The model under review builds one solid part; all positions refer to its coordinate system, in mm. Face numbers are marked on the shaded views. A direction names the side the tool comes from. Give positions to 0.01 mm unless a question says otherwise; leave off trailing zeros. Order: outer loops, then holes, each group sorted by start corner. A loop starts at its lowest first (then second) coordinate and runs counter-clockwise, first axis right, second up. Notation, with made-up numbers: (70.25, -40) - (114.25, -40) arc R13 cw to (114.25, -24) - close; hole circle Ø11 at (-12, 77.5). An arc over 180 degrees is marked (long way). Use CSV: the item, a comma, the result in double quotes. Start each with the question number.
1. Machinability: for the marked faces 1 and 2, which of the approach directions +Z, -Z, +X, -X, +Y, -Y give a long, thin tool a straight path to every point of the face, cutting with its end or side? Answer none if there is none.
2. Take a section at A-A, the plane x = 0. State the section outline as (y, z) points.
3. For pin 1 (2 mm diameter, centred on y = 4, z = 2, fed in from +X), flat-tipped, find the tip position at first contact; note if it passes through.
4. Take a section at D-D, the plane y = 4.85. State the section outline as (x, z) points, then the cut area to 3 significant figures.
5. To check wall thickness, follow line 1 (Y direction, x = 1.25, z = 2.5); line 2 (X direction, y = 4.3, z = 0). State the ranges of each line that lie inside material, in increasing order. Write a range as [from, to].
6. Take a section at C-C, the plane z = 0. State the section outline as (x, y) points.
7. Take a section at B-B, the plane y = 1.7. State the section outline as (x, z) points.
8. Draft analysis for pull direction Z (two halves, no side actions). For the marked faces 3, 4 and 5, state which applies: released by +Z, released by -Z, zero draft, split by the parting line, or undercut.
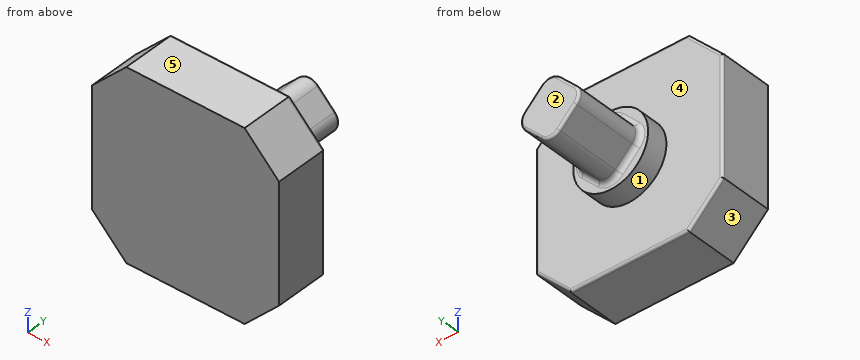
```python
from build123d import *

# Parameters (mm, degrees)
BOSS_EXTRUDE1_DEPTH = 2.14
FILLET1_R           = 0.1
SKETCH2_R           = 1.5
BOSS_EXTRUDE2_DEPTH = 0.86
BOSS_EXTRUDE3_DEPTH = 2.86
FILLET2_R           = 0.1
FILLET3_R           = 0.2


with BuildPart() as part:
    # Sketch1 → Boss-Extrude1 (new body)
    with BuildSketch(Plane(origin=(0, 0, 0), x_dir=(1, 0, 0), z_dir=(0, 1, 0))):
        Polygon((2.371141777, -3.75), (3.75, -2.371141777), (3.75, 2.371141777), (2.371141777, 3.75), (-2.371141777, 3.75), (-3.75, 2.371141777), (-3.75, -2.371141777), (-2.371141777, -3.75), align=None)
    extrude(amount=BOSS_EXTRUDE1_DEPTH)

    # Fillet1
    fillet1_edges = [part.edges().sort_by_distance(p)[0] for p in [
        (3.75, 2.14, 0),
        (3.060570888, 2.14, -3.060570888),
        (0, 2.14, -3.75),
        (-3.060570888, 2.14, -3.060570888),
        (-3.75, 2.14, 0),
        (-3.060570888, 2.14, 3.060570888),
        (0, 2.14, 3.75),
        (3.060570888, 2.14, 3.060570888),
    ]]
    fillet(fillet1_edges, radius=FILLET1_R)

    # Sketch2 → Boss-Extrude2 (add)
    with BuildSketch(Plane(origin=(0, 2.14, 0), x_dir=(1, 0, 0), z_dir=(0, 1, 0))):
        Circle(SKETCH2_R)
    extrude(amount=BOSS_EXTRUDE2_DEPTH)

    # Sketch3 → Boss-Extrude3 (add)
    with BuildSketch(Plane(origin=(0, 3, 0), x_dir=(1, 0, 0), z_dir=(0, 1, 0))):
        with BuildLine():
            Line((-0.353553391, 1.025304833), (-1.025304833, 0.353553391))
            ThreePointArc((-1.025304833, 0.353553391), (-1.171751442, 0), (-1.025304833, -0.353553391))
            Line((-1.025304833, -0.353553391), (-0.353553391, -1.025304833))
            ThreePointArc((-0.353553391, -1.025304833), (0, -1.171751442), (0.353553391, -1.025304833))
            Line((0.353553391, -1.025304833), (1.025304833, -0.353553391))
            ThreePointArc((1.025304833, -0.353553391), (1.171751442, 0), (1.025304833, 0.353553391))
            Line((1.025304833, 0.353553391), (0.353553391, 1.025304833))
            ThreePointArc((0.353553391, 1.025304833), (0, 1.171751442), (-0.353553391, 1.025304833))
        make_face()
    extrude(amount=BOSS_EXTRUDE3_DEPTH)

    # Fillet2
    fillet2_edges = [part.edges().sort_by_distance(p)[0] for p in [
        (-1.171751442, 5.86, 0),
        (-0.689429112, 5.86, 0.689429112),
        (0, 5.86, 1.171751442),
        (0.689429112, 5.86, 0.689429112),
        (1.171751442, 5.86, 0),
        (0.689429112, 5.86, -0.689429112),
        (0, 5.86, -1.171751442),
        (-0.689429112, 5.86, -0.689429112),
    ]]
    fillet(fillet2_edges, radius=FILLET2_R)

    # Fillet3
    fillet3_edges = [part.edges().sort_by_distance(p)[0] for p in [
        (-1.171751442, 3, 0),
        (-0.689429112, 3, 0.689429112),
        (0, 3, 1.171751442),
        (0.689429112, 3, 0.689429112),
        (1.171751442, 3, 0),
        (0.689429112, 3, -0.689429112),
        (0, 3, -1.171751442),
        (-0.689429112, 3, -0.689429112),
    ]]
    fillet(fillet3_edges, radius=FILLET3_R)


solid = part.part
```
Determined:
1,face 1,"+Y"
1,face 2,"+Z, -Z, +X, -X, +Y"
2,outline,"(0, -3.75) - (2.04, -3.75) arc R0.1 ccw to (2.14, -3.65) - (2.14, -1.5) - (3, -1.5) - (3, -1.37) arc R0.2 cw to (3.2, -1.17) - (5.76, -1.17) arc R0.1 ccw to (5.86, -1.07) - (5.86, 1.07) arc R0.1 ccw to (5.76, 1.17) - (3.2, 1.17) arc R0.2 cw to (3, 1.37) - (3, 1.5) - (2.14, 1.5) - (2.14, 3.65) arc R0.1 ccw to (2.04, 3.75) - (0, 3.75) - close"
3,pin 1,"stops at x = 0.38"
4,outline,"(-1.03, -0.35) - (-0.35, -1.03) arc R0.5 ccw to (0.35, -1.03) - (1.03, -0.35) arc R0.5 ccw to (1.03, 0.35) - (0.35, 1.03) arc R0.5 ccw to (-0.35, 1.03) - (-1.03, 0.35) arc R0.5 ccw to start"
4,area,"3.59 mm²"
5,line 1,"y = [0, 2.14]"
5,line 2,"x = [-1.17, 1.17]"
6,outline,"(-3.75, 0) - (3.75, 0) - (3.75, 2.04) arc R0.1 ccw to (3.65, 2.14) - (1.5, 2.14) - (1.5, 3) - (1.37, 3) arc R0.2 cw to (1.17, 3.2) - (1.17, 5.76) arc R0.1 ccw to (1.07, 5.86) - (-1.07, 5.86) arc R0.1 ccw to (-1.17, 5.76) - (-1.17, 3.2) arc R0.2 cw to (-1.37, 3) - (-1.5, 3) - (-1.5, 2.14) - (-3.65, 2.14) arc R0.1 ccw to (-3.75, 2.04) - close"
7,outline,"(-3.75, -2.37) - (-2.37, -3.75) - (2.37, -3.75) - (3.75, -2.37) - (3.75, 2.37) - (2.37, 3.75) - (-2.37, 3.75) - (-3.75, 2.37) - close"
8,face 3,"released by -Z"
8,face 4,"zero draft"
8,face 5,"released by +Z"
